Part model, mm, in its own coordinate system. A direction names the side the tool comes from. Give positions to 0.01 mm unless a question says otherwise; leave off trailing zeros. Order: outer loops, then holes, each group sorted by start corner. A loop starts at its lowest first (then second) coordinate and runs counter-clockwise, first axis right, second up. Notation, with made-up numbers: M 70,-36.5 L 93,-36.5 A25 cw 93,-0.5 Z; hole C -2,56 d5. An arc over 180 degrees is marked long. Return JSON: item names as keys, results as strings.
from build123d import *

# Parameters (mm, degrees)
BOSS_EXTRUDE1_DEPTH      = 82
BOSS_EXTRUDE1_DEPTH_BACK = 153
SKETCH3_W                = 16
SKETCH3_H                = 3
BOSS_EXTRUDE3_DEPTH      = 15
CHAMFER1_SIZE            = 10
SKETCH4_R                = 1.25
CUT_EXTRUDE1_DEPTH       = 10
SKETCH2_R                = 3
CUT_EXTRUDE2_DEPTH       = 10


with BuildPart() as part:
    # Sketch1 → Boss-Extrude1 (new, two sides: drawn at the far end of the back side and taken through both)
    with BuildSketch(Plane.XY.offset(-BOSS_EXTRUDE1_DEPTH_BACK)):
        Polygon((-32.5, 13), (-32.5, 1.5), (-35.5, 1.5), (-35.5, 26.5), (-35.5, 66.5), (-32.5, 66.5), (-32.5, 26.5), (32.5, 26.5), (32.5, 66.5), (35.5, 66.5), (35.5, 26.5), (35.5, 1.5), (32.5, 1.5), (32.5, 13), (30, 13), (30, 23.5), (-30, 23.5), (-30, 13), align=None)
    extrude(amount=BOSS_EXTRUDE1_DEPTH + BOSS_EXTRUDE1_DEPTH_BACK)

    # Sketch3 → Boss-Extrude3 (add)
    with BuildSketch(Plane(origin=(0, 26.5, 0), x_dir=(1, 0, 0), z_dir=(0, 1, 0))):
        with Locations((-19.25, -80.5)):
            Rectangle(SKETCH3_W, SKETCH3_H)
        with Locations((19.25, -80.5)):
            Rectangle(SKETCH3_W, SKETCH3_H)
    extrude(amount=BOSS_EXTRUDE3_DEPTH)

    # Chamfer1
    chamfer1_edges = [part.edges().sort_by_distance(p)[0] for p in [
        (-19.25, 26.5, 79),
        (19.25, 26.5, 79),
    ]]
    chamfer(chamfer1_edges, length=CHAMFER1_SIZE)

    # Sketch4 → Cut-Extrude1 (cut)
    with BuildSketch(Plane.XY.offset(82)):
        with Locations((-14, 33.95)):
            Circle(SKETCH4_R)
        with Locations((14, 33.95)):
            Circle(SKETCH4_R)
    extrude(amount=-CUT_EXTRUDE1_DEPTH, mode=Mode.SUBTRACT)

    # Sketch2 → Cut-Extrude2 (cut)
    with BuildSketch(Plane(origin=(0, 26.5, 0), x_dir=(1, 0, 0), z_dir=(0, 1, 0))):
        with Locations(Location((-25, 128, 0), (0, 0, 270))):
            Circle(SKETCH2_R)
        with Locations(Location((25, 128, 0), (0, 0, 270))):
            Circle(SKETCH2_R)
        with Locations(Location((25, -12, 0), (0, 0, 270))):
            Circle(SKETCH2_R)
        with Locations(Location((-25, -12, 0), (0, 0, 270))):
            Circle(SKETCH2_R)
    extrude(amount=-CUT_EXTRUDE2_DEPTH, mode=Mode.SUBTRACT)


solid = part.part
Q1. Probe line 1 along X through (y, z) = (24, -128); line 2 along X through (y, z) = (28.5, 15.5); line 3 along X through (y, z) = (13.5, -56). List the from-to ranges inside material, lowest first.
Established:
{"line 1": "x = -35.5 to -28, -22 to 22, 28 to 35.5", "line 2": "x = -35.5 to -32.5, 32.5 to 35.5", "line 3": "x = -35.5 to -30, 30 to 35.5"}
Q2. Band-saw the part on B-B (z = -128). Give the cut face in (x, y), then the cut area to 4 significant figures.
Established:
{"outline": "M -35.5,1.5 L -32.5,1.5 L -32.5,13 L -30,13 L -30,23.5 L -28,23.5 L -28,26.5 L -32.5,26.5 L -32.5,66.5 L -35.5,66.5 Z; M -22,23.5 L 22,23.5 L 22,26.5 L -22,26.5 Z; M 28,23.5 L 30,23.5 L 30,13 L 32.5,13 L 32.5,1.5 L 35.5,1.5 L 35.5,66.5 L 32.5,66.5 L 32.5,26.5 L 28,26.5 Z", "area": "601.5 mm²"}
Q3. Two-plate mould, pull along X, no slides. Class faces 5 (the flat face through (-27.25, 32, 78)), 6 (the flat face through (35.5, 34, -37)), 7 (the flat face through (-35.5, 34, -37)): +X half, -X half, draft (parallel to the pull), parting line (faces both ways), or undercut.
Established:
{"face 5": "undercut", "face 6": "+X half", "face 7": "-X half"}
Q4. 3-axis set-ups, long thin cutter, end or side, ignore diameter. For faces 1 (the flat face through (32.5, 7, -37)), 2 (the flat face through (11.25, 32, 78)), 3 (the flat face through (0, 26.5, -37)), 4 (the cylindrical face through (-25, 25, 9)): which of +Z, -Z, +X, -X, +Y, -Y reach the whole face in a straight line?
Established:
{"face 1": "+Z, -Z, -Y", "face 2": "+Z, -Z, +Y", "face 3": "-Z, +Y", "face 4": "+Y, -Y"}
Q5. Pin check, flat tips, straight feed: pin 1 (8 mm diameter, centred on x = -6.5, z = -70.5, fed in from +Y); pin 2 (2 mm diameter, centred on x = -14, y = 33.95, fed in from -Z); pin 3 (2 mm diameter, centred on x = -31, z = -74.5, fed in from -Y); pin 4 (1.5 mm diameter, centred on x = -14, z = 25.5, fed in from -Y). Stop position of each tip, or through.
Established:
{"pin 1": "stops at y = 26.5", "pin 2": "passes through", "pin 3": "stops at y = 13", "pin 4": "stops at y = 23.5"}
Q6. Band-saw the part on C-C (x = 25). Give the cut face in (y, z).
Established:
{"outline": "M 23.5,-153 L 26.5,-153 L 26.5,-131 L 23.5,-131 Z; M 23.5,-125 L 26.5,-125 L 26.5,9 L 23.5,9 Z; M 23.5,15 L 26.5,15 L 26.5,69 L 36.5,79 L 41.5,79 L 41.5,82 L 23.5,82 Z"}
Q7. Band-saw the part on A-A (y = 58). Give the cut face in (x, z).
Established:
{"outline": "M -35.5,-153 L -32.5,-153 L -32.5,82 L -35.5,82 Z; M 32.5,-153 L 35.5,-153 L 35.5,82 L 32.5,82 Z"}
Q8. Band-saw the part on D-D (z = 28). Give the cut face in (x, y), then the cut area to 4 significant figures.
Established:
{"outline": "M -35.5,1.5 L -32.5,1.5 L -32.5,13 L -30,13 L -30,23.5 L 30,23.5 L 30,13 L 32.5,13 L 32.5,1.5 L 35.5,1.5 L 35.5,66.5 L 32.5,66.5 L 32.5,26.5 L -32.5,26.5 L -32.5,66.5 L -35.5,66.5 Z", "area": "637.5 mm²"}
